Answer from the drawing. Dimensions are ordinates in mm from the lowest x, y and z of the part. A direction names the side the tool comes from. Give positions to 0.01 mm unless a question says otherwise; leave off trailing zeros. Order: outer loops, then holes, each group sorted by start corner. A loop starts at its lowest first (then second) coordinate and runs counter-clockwise, first axis right, second up. Notation, with made-up numbers: (52, 9.25) - (61, 9.25) arc R20 ccw to (61, 25.25) - close; hole circle Ø1 at (56, 78). An arc over 180 degrees is marked (long way). Use a Markdown table: item, result. Add a question column.
1) Find section B-B, the plane y = 2.6. Determine the outline of the cut face in (x, z).
2) Find section A-A, the plane x = 4.1. Determine the outline of the cut face in (y, z), plus the area to 3 significant figures.
3) Flat-ended cylindrical pins translate along their axes: pin 1 (3 mm diameter, centred on x = 3, z = 15.5, fed in from -Y); pin 2 (4 mm diameter, centred on x = 1.5, z = 6.5, fed in from +Y). Find the tip coordinate at first contact, or state that the pin passes through.
4) Find section C-C, the plane z = 13.25. Determine the outline of the cut face in (x, y).
5) For the marked faces 1 and 2, determine the directions among +Z, -Z, +X, -X, +Y, -Y from which every point of the face is accessible in a straight line to the end or side of a thin tool.
6) Straight lines are drawn through the part: line 1 (Z direction, x = 3.25, y = 4.4); line 2 (Z direction, x = 7.5, y = 3.55); line 3 (X direction, y = 3.9, z = 14.25). For each, find the intervals that lie inside material, in ascending order.
7) Find section D-D, the plane x = 5.75. Determine the outline of the cut face in (y, z).
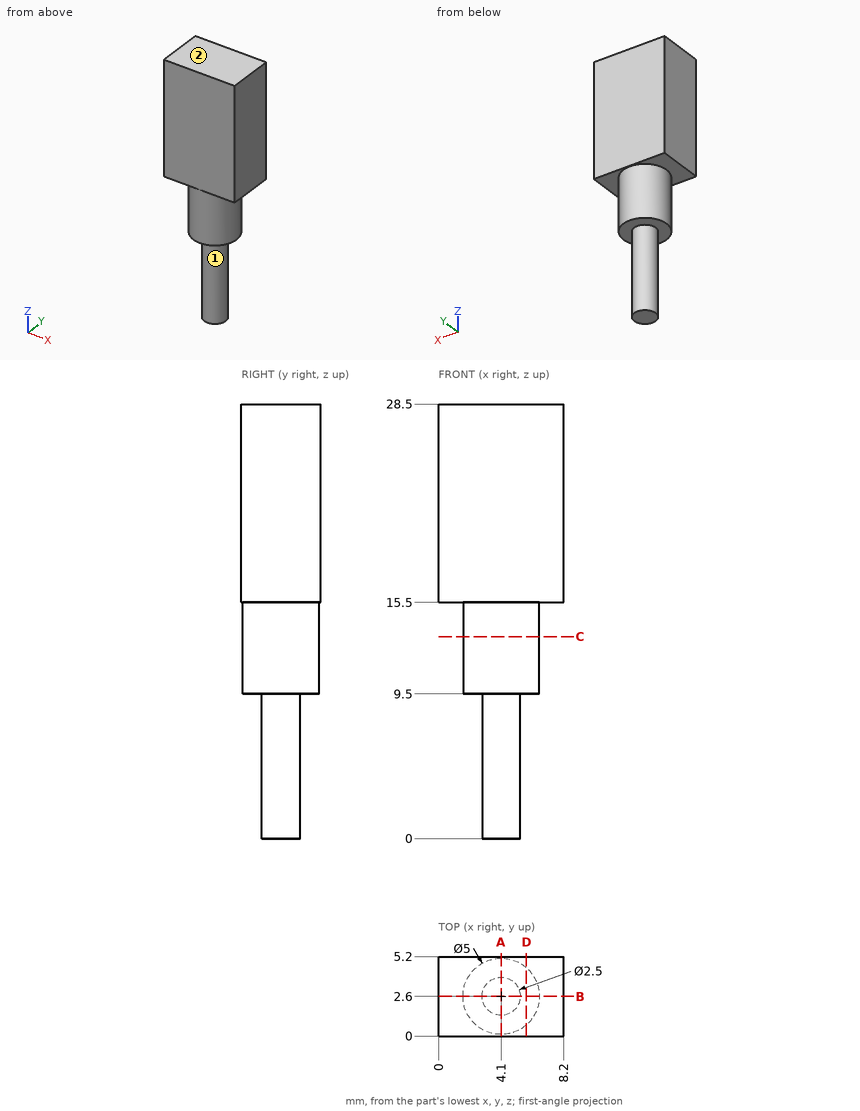
The answers:
| question | item | result |
|---|---|---|
| 1 | outline | (0, 15.5) - (1.6, 15.5) - (1.6, 9.5) - (2.85, 9.5) - (2.85, 0) - (5.35, 0) - (5.35, 9.5) - (6.6, 9.5) - (6.6, 15.5) - (8.2, 15.5) - (8.2, 28.5) - (0, 28.5) - close |
| 2 | outline | (0, 15.5) - (0.1, 15.5) - (0.1, 9.5) - (1.35, 9.5) - (1.35, 0) - (3.85, 0) - (3.85, 9.5) - (5.1, 9.5) - (5.1, 15.5) - (5.2, 15.5) - (5.2, 28.5) - (0, 28.5) - close |
| 2 | area | 121 mm2 |
| 3 | pin 1 | y = 0 |
| 3 | pin 2 | y = 3.7 |
| 4 | outline | circle Ø5 at (4.1, 2.6) |
| 5 | face 1 | -Z |
| 5 | face 2 | +Z, +X, -X, +Y, -Y |
| 6 | line 1 | 9.5 to 28.5 |
| 6 | line 2 | 15.5 to 28.5 |
| 6 | line 3 | 1.96 to 6.24 |
| 7 | outline | (0, 15.5) - (0.72, 15.5) - (0.72, 9.5) - (4.48, 9.5) - (4.48, 15.5) - (5.2, 15.5) - (5.2, 28.5) - (0, 28.5) - close |
